```python
from build123d import *

# Parameters (mm, degrees)
SKETCH_1_R      = 16.5
EXTRUDE_1_DEPTH = 16


with BuildPart() as part:
    # Sketch 1 → Extrude 1 (new body)
    with BuildSketch(Plane(origin=(0, 0, 0), x_dir=(1, 0, 0), z_dir=(0, 1, 0))):
        Circle(SKETCH_1_R)
        with BuildLine():
            ThreePointArc((3, -16.22498074), (0, -16.5), (-3, -16.22498074))
            Line((-3, -16.22498074), (-3, -17.748239349))
            ThreePointArc((-3, -17.748239349), (0, -18), (3, -17.748239349))
            Line((3, -17.748239349), (3, -16.22498074))
        make_face()
        with BuildLine():
            Line((11.472195886, -13.870426149), (10.710566581, -12.551245496))
            ThreePointArc((10.710566581, -12.551245496), (8.25, -14.289419162), (5.514414158, -15.551245496))
            Line((5.514414158, -15.551245496), (6.276043463, -16.870426149))
            ThreePointArc((6.276043463, -16.870426149), (9, -15.588457268), (11.472195886, -13.870426149))
        make_face()
        with BuildLine():
            Line((16.870426149, -6.276043463), (15.551245496, -5.514414158))
            ThreePointArc((15.551245496, -5.514414158), (14.289419162, -8.25), (12.551245496, -10.710566581))
            Line((12.551245496, -10.710566581), (13.870426149, -11.472195886))
            ThreePointArc((13.870426149, -11.472195886), (15.588457268, -9), (16.870426149, -6.276043463))
        make_face()
        with BuildLine():
            Line((17.748239349, 3), (16.22498074, 3))
            ThreePointArc((16.22498074, 3), (16.431101336, 1.506289779), (16.5, 0))
            ThreePointArc((16.5, 0), (16.431101336, -1.506289779), (16.22498074, -3))
            Line((16.22498074, -3), (17.748239349, -3))
            ThreePointArc((17.748239349, -3), (18, 0), (17.748239349, 3))
        make_face()
        with BuildLine():
            Line((13.870426149, 11.472195886), (12.551245496, 10.710566581))
            ThreePointArc((12.551245496, 10.710566581), (14.289419162, 8.25), (15.551245496, 5.514414158))
            Line((15.551245496, 5.514414158), (16.870426149, 6.276043463))
            ThreePointArc((16.870426149, 6.276043463), (15.588457268, 9), (13.870426149, 11.472195886))
        make_face()
        with BuildLine():
            Line((6.276043463, 16.870426149), (5.514414158, 15.551245496))
            ThreePointArc((5.514414158, 15.551245496), (8.25, 14.289419162), (10.710566581, 12.551245496))
            Line((10.710566581, 12.551245496), (11.472195886, 13.870426149))
            ThreePointArc((11.472195886, 13.870426149), (9, 15.588457268), (6.276043463, 16.870426149))
        make_face()
        with BuildLine():
            ThreePointArc((3, 17.748239349), (0, 18), (-3, 17.748239349))
            Line((-3, 17.748239349), (-3, 16.22498074))
            ThreePointArc((-3, 16.22498074), (0, 16.5), (3, 16.22498074))
            Line((3, 16.22498074), (3, 17.748239349))
        make_face()
        with BuildLine():
            ThreePointArc((-10.710566581, 12.551245496), (-8.25, 14.289419162), (-5.514414158, 15.551245496))
            Line((-5.514414158, 15.551245496), (-6.276043463, 16.870426149))
            ThreePointArc((-6.276043463, 16.870426149), (-9, 15.588457268), (-11.472195886, 13.870426149))
            Line((-11.472195886, 13.870426149), (-10.710566581, 12.551245496))
        make_face()
        with BuildLine():
            ThreePointArc((-15.551245496, 5.514414158), (-14.289419162, 8.25), (-12.551245496, 10.710566581))
            Line((-12.551245496, 10.710566581), (-13.870426149, 11.472195886))
            ThreePointArc((-13.870426149, 11.472195886), (-15.588457268, 9), (-16.870426149, 6.276043463))
            Line((-16.870426149, 6.276043463), (-15.551245496, 5.514414158))
        make_face()
        with BuildLine():
            ThreePointArc((-16.22498074, -3), (-16.5, 0), (-16.22498074, 3))
            Line((-16.22498074, 3), (-17.748239349, 3))
            ThreePointArc((-17.748239349, 3), (-18, 0), (-17.748239349, -3))
            Line((-17.748239349, -3), (-16.22498074, -3))
        make_face()
        with BuildLine():
            ThreePointArc((-12.551245496, -10.710566581), (-14.289419162, -8.25), (-15.551245496, -5.514414158))
            Line((-15.551245496, -5.514414158), (-16.870426149, -6.276043463))
            ThreePointArc((-16.870426149, -6.276043463), (-15.588457268, -9), (-13.870426149, -11.472195886))
            Line((-13.870426149, -11.472195886), (-12.551245496, -10.710566581))
        make_face()
        with BuildLine():
            ThreePointArc((-5.514414158, -15.551245496), (-8.25, -14.289419162), (-10.710566581, -12.551245496))
            Line((-10.710566581, -12.551245496), (-11.472195886, -13.870426149))
            ThreePointArc((-11.472195886, -13.870426149), (-9, -15.588457268), (-6.276043463, -16.870426149))
            Line((-6.276043463, -16.870426149), (-5.514414158, -15.551245496))
        make_face()
    extrude(amount=EXTRUDE_1_DEPTH)


solid = part.part
```
Input: part model. Units: mm. Frame: model coordinates. A direction names the side the tool comes from. Round coordinates to 2 decimals unless told otherwise and drop trailing zeros. Write each loop counter-clockwise with the first axis right and the second up, starting at its lowest first coordinate (ties: lowest second). Pieces come first, ordered by that corner, then holes. Notation, with made-up numbers: (87.5, 10.25) - (116.5, 10.25) arc R16 cw to (116.5, 14.25) - close; hole circle Ø9 at (-26.5, 12). An arc over 180 degrees is marked (long way). Write item = value, one per line.
(1) Contact query for flat-ended pins moving along their axis: pin 1 Ø0.8 at (y, z) = (6, 17) entering from -X; pin 2 Ø4 at (x, y) = (7, 2) entering from +Z; pin 3 Ø3 at (y, z) = (13, 10) entering from +X. Output: stop coordinate, or through.
Geometry check:
pin_1 = -6.96
pin_2 = 16.87
pin_3 = 15.87
(2) Pull-direction query (X, two-part tool) for faces 1 (the cylindrical face through (15.942, 7.888, -4.253)), 2 (the cylindrical face through (-15.567, 7.888, -9.037)), 3 (the cylindrical face through (4.288, 7.888, -15.933)); classes: +X half, -X half, draft (parallel to the pull), parting line (faces both ways), or undercut.
Geometry check:
face_1 = +X half
face_2 = -X half
face_3 = undercut
(3) Access query for faces 4 (the flat face through (-13.202, 7.888, -11.086)), 5 (the cylindrical face through (4.253, 7.888, 15.942)), 6 (the flat face through (11.097, 7.888, 13.22)). Directions: +Z, -Z, +X, -X, +Y, -Y. A direction counts if a zero-diameter tool reaches every point of the face in a straight line with its end or side. Return the directions, or none.
Geometry check:
face_4 = -Z, +Y, -Y
face_5 = +Z, +Y, -Y
face_6 = +X, +Y, -Y
(4) Section query A-A on x = 10. Output: boundary loops of the cut face in (y, z), then the cut area to 3 significant figures.
Geometry check:
outline = (0, -14.97) - (16, -14.97) - (16, 14.97) - (0, 14.97) - close
area = 479 mm^2
(5) Material intervals for probe 1 along Z at (x, y) = (11, 6.25); probe 2 along X at (y, z) = (5.25, 8); probe 3 along X at (y, z) = (7.5, -12), sorted ascending.
Geometry check:
probe_1 = -14.25 to -13.05, -12.3 to 12.3, 13.05 to 14.25
probe_2 = -16.12 to 16.12
probe_3 = -11.32 to 11.32
(6) Section query B-B on z = 5. Output: boundary loops of the cut face in (x, y), then the cut area to 3 significant figures.
Geometry check:
outline = (-15.72, 0) - (15.72, 0) - (15.72, 16) - (-15.72, 16) - close
area = 503 mm^2
